Verification items for the finished model (mm, model axes). A direction names the side the tool comes from. Round coordinates to 2 decimals unless told otherwise and drop trailing zeros. Order: outer loops, then holes, each group sorted by start corner. A loop starts at its lowest first (then second) coordinate and runs counter-clockwise, first axis right, second up. Notation, with made-up numbers: M -15.5,-39 L 10.5,-39 A33 ccw 10.5,-3 Z; hole C -19,-0.5 d10. An arc over 180 degrees is marked long. Return JSON: item names as keys, results as strings. Group by question number.
from build123d import *

# Parameters (mm, degrees)
SKETCH1_R           = 37.5
BOSS_EXTRUDE1_DEPTH = 1.5
SKETCH4_R           = 7.25
BOSS_EXTRUDE2_DEPTH = 6
SKETCH5_R           = 5.5
CUT_EXTRUDE2_DEPTH  = 7
SKETCH8_R           = 2.75
SKETCH8_R_2         = 1.65
CUT_EXTRUDE3_DEPTH  = 10
CUT_EXTRUDE5_DEPTH  = 5


with BuildPart() as part:
    # Sketch1 → Boss-Extrude1 (new body)
    with BuildSketch(Plane(origin=(0, 0, 0), x_dir=(1, 0, 0), z_dir=(0, 1, 0))):
        with Locations(Location((0, 0, 0), (0, 0, 270))):
            Circle(SKETCH1_R)
    extrude(amount=BOSS_EXTRUDE1_DEPTH)

    # Sketch4 → Boss-Extrude2 (add)
    with BuildSketch(Plane.XZ):
        with Locations(Location((0, 0, 0), (0, 0, 270))):
            Circle(SKETCH4_R)
    extrude(amount=BOSS_EXTRUDE2_DEPTH)

    # Sketch5 → Cut-Extrude2 (cut)
    with BuildSketch(Plane.XZ.offset(6)):
        with Locations(Location((0, 0, 0), (0, 0, 270))):
            Circle(SKETCH5_R)
    extrude(amount=-CUT_EXTRUDE2_DEPTH, mode=Mode.SUBTRACT)

    # Sketch8 → Cut-Extrude3 (cut)
    with BuildSketch(Plane(origin=(0, 1.5, 0), x_dir=(1, 0, 0), z_dir=(0, 1, 0))):
        with Locations(Location((-23.416394486, 23.949580961, 0), (0, 0, 270))):
            Circle(SKETCH8_R)
        with Locations(Location((23.949580961, 23.416394486, 0), (0, 0, 270))):
            Circle(SKETCH8_R)
        with Locations(Location((23.416394486, -23.949580961, 0), (0, 0, 270))):
            Circle(SKETCH8_R)
        with Locations(Location((-23.949580961, -23.416394486, 0), (0, 0, 270))):
            Circle(SKETCH8_R)
        with Locations(Location((-30.519872414, -12.551389877, 0), (0, 0, 270))):
            Circle(SKETCH8_R_2)
        with Locations(Location((-12.551389877, 30.519872414, 0), (0, 0, 270))):
            Circle(SKETCH8_R_2)
        with Locations(Location((30.519872414, 12.551389878, 0), (0, 0, 270))):
            Circle(SKETCH8_R_2)
        with Locations(Location((12.551389878, -30.519872414, 0), (0, 0, 270))):
            Circle(SKETCH8_R_2)
    extrude(amount=-CUT_EXTRUDE3_DEPTH, mode=Mode.SUBTRACT)

    # Sketch9 → Cut-Extrude5 (cut, symmetric)
    with BuildSketch(Plane(origin=(0, 1.5, 0), x_dir=(1, 0, 0), z_dir=(0, 1, 0))):
        with BuildLine():
            Line((15.152911059, 1.700080088), (13.450685177, -8.316302683))
            Line((13.450685177, -8.316302683), (27.023681414, -10.622954298))
            ThreePointArc((27.023681414, -10.622954298), (27.636041802, -16.917145139), (29.657895546, -22.909134042))
            ThreePointArc((29.657895546, -22.909134042), (42.084378473, -8.529589687), (36.242968745, 9.555395969))
            ThreePointArc((36.242968745, 9.555395969), (32.067942495, 4.855826196), (29.0581189, -0.663028953))
            Line((29.0581189, -0.663028953), (15.152911059, 1.700080088))
        make_face()
    extrude(amount=CUT_EXTRUDE5_DEPTH, both=True, mode=Mode.SUBTRACT)


solid = part.part
1. Access from +Z, -Z, +X, -X, +Y, -Y to the whole of each face (thin tool, end or side, straight path). Record for faces 5 (the face through (27.618, 0.76, 16.83)), 6 (the face through (0, 1.5, -1)), 7 (the face through (14.314, 0.76, 3.238)), 8 (the face through (-5.37, -2.55, 1.19)).
2. Go/stop test with flat-tipped pins: pin 1 (2 mm diameter, centred on y = 0.5, z = 14.5, fed in from +X); pin 2 (5.5 mm diameter, centred on x = 0, z = -1, fed in from -Y); pin 3 (1 mm diameter, centred on x = 1.5, z = -8.5, fed in from -Y); pin 4 (2 mm diameter, centred on x = -12.55, z = -30.52, fed in from +Y). Record where each tip stops, or that it passes through.
3. Cross-section at A-A (y = -2.25). Enter the section's corners in (x, z), plus the area to 3 significant figures.
4. Cross-section at B-B (x = 0). Enter the section's corners in (y, z).
5. Thickness scan on line 1 along Y through (x, z) = (-20, -29); line 2 along Y through (x, z) = (-3.5, 2.5); line 3 along X through (y, z) = (-3.75, 2.5). Record the ranges inside material, lowest first. Write a range as from..to.
6. Draft check along X on faces 1 (the face through (-25, 0.76, 25.96)), 2 (the face through (5, -6, -3)), 3 (the face through (-36.45, 0.74, -8.82)), 4 (the face through (0, 1, 0)). Enter one of: +X half, -X half, draft (parallel to the pull), parting line (faces both ways), or undercut.
Computed:
{
 "1": {"face 5": "+X, +Y, -Y", "face 6": "+Z, -Z, +X, -X, +Y", "face 7": "+Y, -Y", "face 8": "-Y"},
 "2": {"pin 1": "stops at x = 27.37", "pin 2": "stops at y = 1", "pin 3": "stops at y = 0", "pin 4": "passes through"},
 "3": {"outline": "C 0,0 d14.5; hole C 0,0 d11", "area": "70.1 mm²"},
 "4": {"outline": "M -6,-7.25 L 0,-7.25 L 0,-37.5 L 1.5,-37.5 L 1.5,37.5 L 0,37.5 L 0,7.25 L -6,7.25 L -6,5.5 L 1,5.5 L 1,-5.5 L -6,-5.5 Z"},
 "5": {"line 1": "y = 0..1.5", "line 2": "y = 1..1.5", "line 3": "x = -6.81..-4.9, 4.9..6.81"},
 "6": {"face 1": "undercut", "face 2": "draft", "face 3": "parting line", "face 4": "undercut"}
}
